Can you work these out from the drawing? Everything is in mm from the part's minimum corner. A direction names the side the tool comes from. Round coordinates to 2 decimals unless told otherwise and drop trailing zeros. Loops run counter-clockwise (first coordinate to the right, second up) from the corner with the lowest first, then second, coordinate; pieces in that order, holes last. Notation, with made-up numbers: (86.25, 37.5) -> (122.25, 37.5) arc R13 cw to (122.25, 57.5) -> close; hole circle Ø5 at (82.25, 62). An arc over 180 degrees is marked (long way). Answer as a JSON object with one key per item and string values.
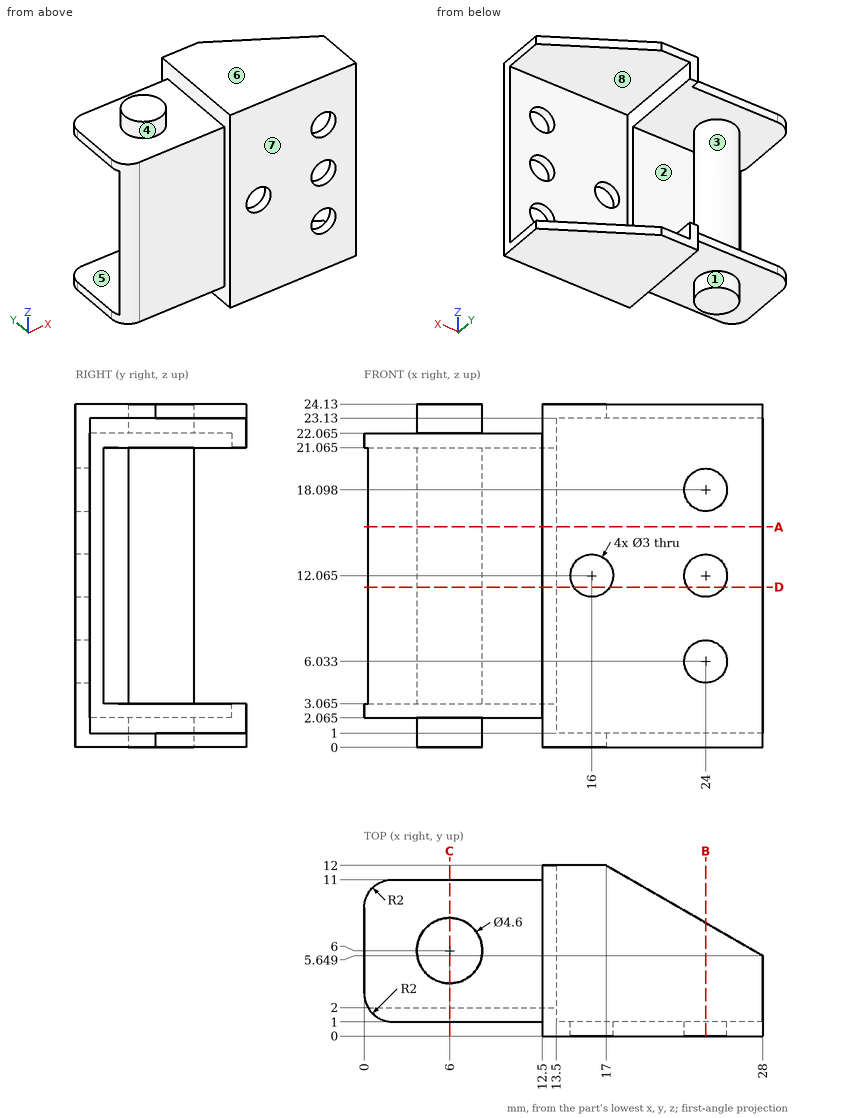
Q1. I want a section at C-C, the plane x = 6. Write out the boundary of the cut face in (y, z) (1 decimal), then the cut area to 3 significant figures.
Determined:
{"outline": "(1, 2.1) -> (3.7, 2.1) -> (3.7, 0) -> (8.3, 0) -> (8.3, 2.1) -> (11, 2.1) -> (11, 3.1) -> (8.3, 3.1) -> (8.3, 21.1) -> (11, 21.1) -> (11, 22.1) -> (8.3, 22.1) -> (8.3, 24.1) -> (3.7, 24.1) -> (3.7, 22.1) -> (1, 22.1) -> close; hole (2, 3.1) -> (3.7, 3.1) -> (3.7, 21.1) -> (2, 21.1) -> close", "area": "140 mm²"}
Q2. I'm going to push flat-ended pins straight in: pin 1 (10.5 mm diameter, centred on x = 5, z = 16, fed in from +Y); pin 2 (2.5 mm diameter, centred on x = 16, z = 12.065, fed in from +Y); pin 3 (2 mm diameter, centred on y = 4, z = 18.5, fed in from +X); pin 4 (3 mm diameter, centred on x = 7, z = 12.5, fed in from -Y). Where does each tip first touch, or does it pass through?
Determined:
{"pin 1": "y = 11", "pin 2": "through", "pin 3": "x = 8.07", "pin 4": "y = 1"}
Q3. We'd pull the mould along Z, two halves only. Please class the marked faces 5, 6, 7 and 8: pulls with the +Z half, pulls with the -Z half, needs draft (parallel to the pull), parting line crosses it, or undercut.
Determined:
{"face 5": "undercut", "face 6": "pulls with the +Z half", "face 7": "needs draft", "face 8": "undercut"}
Q4. If I drill on L1, parallel to Z at x = 10.5, y = 10.5 (1 decimal); L2, parallel to Z at x = 19.5, y = 2.75; L3, parallel to Y at x = 12.25, z = 9.75, over which ranges is the centre line in solid material (lowest first)? Write a range as [from, to].
Determined:
{"L1": "[2.1, 3.1], [21.1, 22.1]", "L2": "[0, 1], [23.13, 24.13]", "L3": "[1, 2]"}
Q5. I want a section at D-D, the plane z = 11.25. Write out the boundary of the cut face in (x, y).
Determined:
{"outline": "(0.27, 2) arc R2 ccw to (2, 1) -> (12.5, 1) -> (12.5, 0) -> (14.74, 0) -> (14.74, 1) -> (13.5, 1) -> (13.5, 2) -> close; circle Ø4.6 at (6, 6); (17.26, 0) -> (22.74, 0) -> (22.74, 1) -> (17.26, 1) -> close; (25.26, 0) -> (28, 0) -> (28, 1) -> (25.26, 1) -> close"}
Q6. On a 3-axis mill with a long thin cutter (end or side, diameter ignored), from which of +Z, -Z, +X, -X, +Y, -Y can I reach the whole of each face in a straight line? I mean the marked faces 1, 2, 3 and 4. Say none if no direction works.
Determined:
{"face 1": "-Z", "face 2": "+X, -X", "face 3": "none", "face 4": "+Z"}
Q7. I want a section at B-B, the plane x = 24. Write out the boundary of the cut face in (y, z) (1 decimal).
Determined:
{"outline": "(0, 0) -> (8, 0) -> (8, 1) -> (1, 1) -> (1, 4.5) -> (0, 4.5) -> close; (0, 7.5) -> (1, 7.5) -> (1, 10.6) -> (0, 10.6) -> close; (0, 13.6) -> (1, 13.6) -> (1, 16.6) -> (0, 16.6) -> close; (0, 19.6) -> (1, 19.6) -> (1, 23.1) -> (8, 23.1) -> (8, 24.1) -> (0, 24.1) -> close"}
Q8. I want a section at A-A, the plane z = 15.5. Write out the boundary of the cut face in (x, y).
Determined:
{"outline": "(0.27, 2) arc R2 ccw to (2, 1) -> (12.5, 1) -> (12.5, 0) -> (28, 0) -> (28, 1) -> (13.5, 1) -> (13.5, 2) -> close; circle Ø4.6 at (6, 6)"}
